```python
from build123d import *

# Parameters (mm, degrees)
SKETCH1_W           = 750
SKETCH1_H           = 1490
BOSS_EXTRUDE1_DEPTH = 30
SKETCH2_W           = 100
SKETCH2_H           = 100
BOSS_EXTRUDE2_DEPTH = 800


with BuildPart() as part:
    # Sketch1 → Boss-Extrude1 (new body)
    with BuildSketch(Plane(origin=(0, 0, 0), x_dir=(1, 0, 0), z_dir=(0, 1, 0))):
        with Locations((375, 745)):
            Rectangle(SKETCH1_W, SKETCH1_H)
    extrude(amount=BOSS_EXTRUDE1_DEPTH)

    # Sketch2 → Boss-Extrude2 (add)
    with BuildSketch(Plane(origin=(0, 30, 0), x_dir=(1, 0, 0), z_dir=(0, 1, 0))):
        with Locations((50, 50)):
            Rectangle(SKETCH2_W, SKETCH2_H)
        with Locations((700, 50)):
            Rectangle(SKETCH2_W, SKETCH2_H)
        with Locations((700, 1440)):
            Rectangle(SKETCH2_W, SKETCH2_H)
        with Locations((50, 1440)):
            Rectangle(SKETCH2_W, SKETCH2_H)
    extrude(amount=-BOSS_EXTRUDE2_DEPTH)


solid = part.part
```
The listing builds one solid part. Answer for the finished solid, in the listing's coordinates (mm). A direction names the side the tool comes from. Give positions to 0.01 mm unless a question says otherwise; leave off trailing zeros. Order: outer loops, then holes, each group sorted by start corner. A loop starts at its lowest first (then second) coordinate and runs counter-clockwise, first axis right, second up. Notation, with made-up numbers: M 87,24 L 116,24 A3 ccw 116,28 Z; hole C -21,-28.5 d6. An arc over 180 degrees is marked long. Put each result on its own line as item: value. Start each with the question number.
Item 1: Find the intervals of material crossed by line 1 along Z through (x, y) = (683, -432); line 2 along X through (y, z) = (-690.5, -1428.5); line 3 along Y through (x, z) = (580, -782.5), in increasing order.
Item 2: The part is cut by section A-A, the plane y = -424.5. Determine the outline of the cut face in (x, z), and give its area (3 significant figures).
Item 3: For a pull along X with two mould halves and no side action, classify faces 1 (the face through (370, 30, -755)), 2 (the face through (750, 13, -742)), 3 (the face through (650, -380, -49)), 4 (the face through (650, -380, -1439)) as +X half, -X half, draft (parallel to the pull), parting line (faces both ways), or undercut.
Item 4: The part is cut by section D-D, the plane x = 348.5. Determine the outline of the cut face in (y, z).
Item 5: Which of the six approach directions +Z, -Z, +X, -X, +Y, -Y give full straight-line access (tool end or side, diameter ignored) to faces 5 (the face through (699, -380, -1390)), 6 (the face through (49, -770, -51)), 7 (the face through (100, -380, -49))?
Item 6: The part is cut by section C-C, the plane z = -505.5. Determine the outline of the cut face in (x, y), and give its area (3 significant figures).
Item 7: The part is cut by section B-B, the plane x = 73. Determine the outline of the cut face in (y, z), and give its area (3 significant figures).
Item 8: A flat-ended cylindrical pin translates along its axis: P1, Ø1, axis at x = 594, z = -1206.5, coming from the -Y side. Find the tip coordinate at first contact, or state that the pin passes through.
Answer key:
1. line 1: z = -1490 to -1390, -100 to 0
1. line 2: x = 0 to 100, 650 to 750
1. line 3: y = 0 to 30
2. outline: M 0,-1490 L 100,-1490 L 100,-1390 L 0,-1390 Z; M 0,-100 L 100,-100 L 100,0 L 0,0 Z; M 650,-1490 L 750,-1490 L 750,-1390 L 650,-1390 Z; M 650,-100 L 750,-100 L 750,0 L 650,0 Z
2. area: 40,000 mm²
3. face 1: draft
3. face 2: +X half
3. face 3: undercut
3. face 4: undercut
4. outline: M 0,-1490 L 30,-1490 L 30,0 L 0,0 Z
5. face 5: +X, -X, -Y
5. face 6: +Z, -Z, +X, -X, -Y
5. face 7: +Z, -Z, -Y
6. outline: M 0,0 L 750,0 L 750,30 L 0,30 Z
6. area: 22,500 mm²
7. outline: M -770,-1490 L 30,-1490 L 30,0 L -770,0 L -770,-100 L 0,-100 L 0,-1390 L -770,-1390 Z
7. area: 199,000 mm²
8. P1: stops at y = 0
